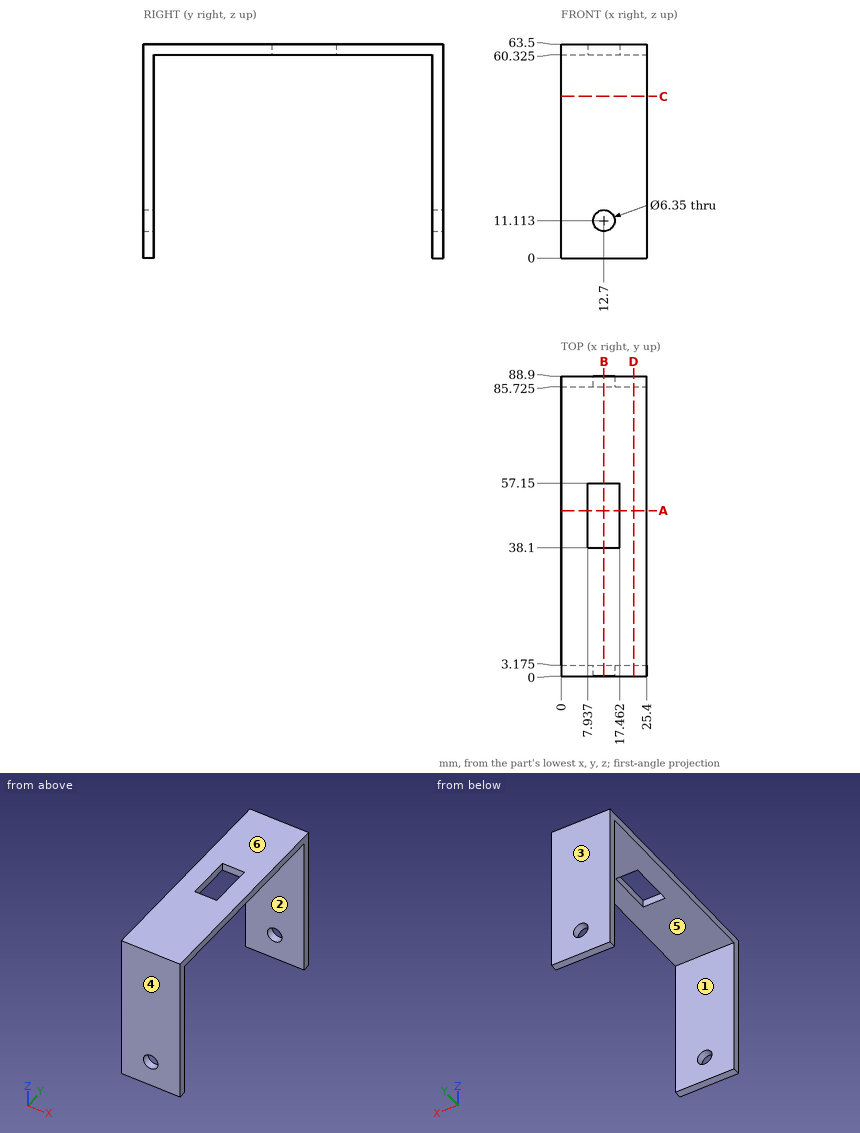
Geometry: see drawing. Coordinates: mm, zero at the bounding-box minimum. A direction names the side the tool comes from. Give positions to 0.01 mm unless a question says otherwise; leave off trailing zeros. Write each loop counter-clockwise with the first axis right and the second up, starting at its lowest first coordinate (ties: lowest second). Pieces come first, ordered by that corner, then holes. Notation, with made-up numbers: M -38,23.5 L -26,23.5 A23 cw -26,33.5 Z; hole C 37.5,10 d3. An arc over 180 degrees is marked long. Answer as a JSON object with one key per item and string values.
Q1. Access query for the marked faces 5 and 6. Directions: +Z, -Z, +X, -X, +Y, -Y. A direction counts if a zero-diameter tool reaches every point of the face in a straight line with its end or side. Return the directions, or none.
Geometry check:
{"face 5": "-Z, +X, -X", "face 6": "+Z, +X, -X, +Y, -Y"}
Q2. Cut plane A-A, the plane y = 49. Return the cut outline in (x, z) (1 decimal).
Geometry check:
{"outline": "M 0,60.3 L 7.9,60.3 L 7.9,63.5 L 0,63.5 Z; M 17.5,60.3 L 25.4,60.3 L 25.4,63.5 L 17.5,63.5 Z"}
Q3. Cut plane D-D, the plane x = 21.5. Return the cut outline in (y, z) (1 decimal).
Geometry check:
{"outline": "M 0,0 L 3.2,0 L 3.2,60.3 L 85.7,60.3 L 85.7,0 L 88.9,0 L 88.9,63.5 L 0,63.5 Z"}
Q4. Contact query for flat-ended pins moving along their axis: P1, Ø10, axis at x = 17, y = 12.5, coming from the -Z side (1 decimal); P2, Ø4, axis at x = 12.7, z = 11.11, coming from the +Y side; P3, Ø10, axis at x = 12.7, z = 11.11, coming from the -Y side. Output: stop coordinate, or through.
Geometry check:
{"P1": "stops at z = 60.3", "P2": "passes through", "P3": "stops at y = 0"}
Q5. Cut plane C-C, the plane z = 48. Return the cut outline in (x, y) (1 decimal).
Geometry check:
{"outline": "M 0,0 L 25.4,0 L 25.4,3.2 L 0,3.2 Z; M 0,85.7 L 25.4,85.7 L 25.4,88.9 L 0,88.9 Z"}
Q6. Cut plane B-B, the plane x = 12.7. Count the separate pieces of the cut face and the enclosed holes in it.
Geometry check:
{"separate pieces": "4", "enclosed holes": "0"}
Q7. Mould query, pull axis Y, two halves, no side actions, for the marked faces 1, 2, 3 and 4. Classes: +Y half, -Y half, draft (parallel to the pull), parting line (faces both ways), or undercut.
Geometry check:
{"face 1": "undercut", "face 2": "undercut", "face 3": "+Y half", "face 4": "-Y half"}
Q8. Ray query, line 1 along Z through (x, y) = (12.7, 0.7); line 2 along Y through (x, z) = (13.5, 43) (1 decimal); line 3 along Z through (x, y) = (14.75, 4) (1 decimal). Return the intervals inside material, ascending.
Geometry check:
{"line 1": "z = 0 to 7.94, 14.29 to 63.5", "line 2": "y = 0 to 3.2, 85.7 to 88.9", "line 3": "z = 60.3 to 63.5"}
